For this review, take the finished solid that the model builds, in its own axes (mm). Give positions to 0.01 mm unless a question says otherwise; leave off trailing zeros. Loops run counter-clockwise (first coordinate to the right, second up) from the corner with the lowest first, then second, coordinate; pieces in that order, holes last.
```python
from build123d import *

# Parameters (mm, degrees)
BOARD_OUTLINE_DEPTH = 1.6
SKETCH2_R           = 1.016
SKETCH2_R_2         = 1.651
SKETCH2_R_3         = 0.254
SKETCH2_R_4         = 0.3
NPTH_DEPTH          = 55.024838732
SKETCH3_R           = 0.51
PTH_DEPTH           = 55.024838732
SKETCH4_W           = 11.674517828
SKETCH4_H           = 37.265337661
CUT_EXTRUDE1_DEPTH  = 10
SKETCH6_W           = 12.562793993
SKETCH6_H           = 36.934833376
CUT_EXTRUDE2_DEPTH  = 10


with BuildPart() as part:
    # Sketch1 → Board_Outline (new body)
    with BuildSketch(Plane.XY):
        Polygon((2.54, 35.56), (38.1, 35.56), (38.7574, 35.473452), (39.37, 35.219705), (39.896051, 34.816051), (40.299705, 34.29), (40.553452, 33.6774), (40.64, 33.02), (40.64, 2.54), (40.553452, 1.8826), (40.299705, 1.27), (39.896051, 0.743949), (39.37, 0.340295), (38.7574, 0.086548), (38.1, 0), (2.54, 0), (1.8826, 0.086548), (1.27, 0.340295), (0.743949, 0.743949), (0.340295, 1.27), (0.086548, 1.8826), (0, 2.54), (0, 33.02), (0.086548, 33.6774), (0.340295, 34.29), (0.743949, 34.816051), (1.27, 35.219705), (1.8826, 35.473452), align=None)
    extrude(amount=BOARD_OUTLINE_DEPTH)

    # Sketch2 → NPTH (cut, through all)
    with BuildSketch(Plane.XY):
        with Locations((20.32, 33.02)):
            Circle(SKETCH2_R)
        with Locations((20.32, 28.448)):
            Circle(SKETCH2_R)
        with Locations((2.54, 33.02)):
            Circle(SKETCH2_R_2)
        with Locations((38.1, 33.02)):
            Circle(SKETCH2_R_2)
        with Locations((2.54, 2.54)):
            Circle(SKETCH2_R_2)
        with Locations((38.1, 2.54)):
            Circle(SKETCH2_R_2)
        with Locations((21.463, 9.525)):
            Circle(SKETCH2_R_3)
        with Locations((27.686, 22.86)):
            Circle(SKETCH2_R_3)
        with Locations((20.955, 14.732)):
            Circle(SKETCH2_R_3)
        with Locations((24.13, 13.335)):
            Circle(SKETCH2_R_3)
        with Locations((24.13, 18.669)):
            Circle(SKETCH2_R_3)
        with Locations((19.304, 20.701)):
            Circle(SKETCH2_R_3)
        with Locations((18.415, 14.986)):
            Circle(SKETCH2_R_3)
        with Locations((16.383, 11.43)):
            Circle(SKETCH2_R_3)
        with Locations((16.571, 9.591)):
            Circle(SKETCH2_R_3)
        with Locations((26.67, 24.13)):
            Circle(SKETCH2_R_3)
        with Locations((26.543, 9.525)):
            Circle(SKETCH2_R_3)
        with Locations((26.924, 10.795)):
            Circle(SKETCH2_R_3)
        with Locations((26.289, 14.605)):
            Circle(SKETCH2_R_3)
        with Locations((21.463, 6.096)):
            Circle(SKETCH2_R_3)
        with Locations((14.605, 29.972)):
            Circle(SKETCH2_R_4)
        with Locations((21.209, 8.128)):
            Circle(SKETCH2_R_3)
        with Locations((27.305, 6.35)):
            Circle(SKETCH2_R_3)
        with Locations((27.432, 12.827)):
            Circle(SKETCH2_R_3)
        with Locations((21.844, 19.304)):
            Circle(SKETCH2_R_3)
        with Locations((21.844, 13.843)):
            Circle(SKETCH2_R_3)
        with Locations((25.4, 30.48)):
            Circle(SKETCH2_R_3)
        with Locations((22.86, 33.02)):
            Circle(SKETCH2_R_3)
    extrude(amount=NPTH_DEPTH, mode=Mode.SUBTRACT)

    # Sketch3 → PTH (cut, through all)
    with BuildSketch(Plane.XY):
        with Locations((11.43, 31.75)):
            Circle(SKETCH3_R)
        with Locations((11.43, 29.21)):
            Circle(SKETCH3_R)
        with Locations((11.43, 26.67)):
            Circle(SKETCH3_R)
        with Locations((34.29, 31.75)):
            Circle(SKETCH3_R)
        with Locations((11.43, 24.13)):
            Circle(SKETCH3_R)
        with Locations((11.43, 21.59)):
            Circle(SKETCH3_R)
        with Locations((11.43, 19.05)):
            Circle(SKETCH3_R)
        with Locations((11.43, 16.51)):
            Circle(SKETCH3_R)
        with Locations((11.43, 13.97)):
            Circle(SKETCH3_R)
        with Locations((11.43, 11.43)):
            Circle(SKETCH3_R)
        with Locations((11.43, 8.89)):
            Circle(SKETCH3_R)
        with Locations((11.43, 6.35)):
            Circle(SKETCH3_R)
        with Locations((11.43, 3.81)):
            Circle(SKETCH3_R)
        with Locations((29.21, 3.81)):
            Circle(SKETCH3_R)
        with Locations((29.21, 6.35)):
            Circle(SKETCH3_R)
        with Locations((29.21, 8.89)):
            Circle(SKETCH3_R)
        with Locations((29.21, 11.43)):
            Circle(SKETCH3_R)
        with Locations((29.21, 13.97)):
            Circle(SKETCH3_R)
        with Locations((29.21, 16.51)):
            Circle(SKETCH3_R)
        with Locations((29.21, 19.05)):
            Circle(SKETCH3_R)
        with Locations((29.21, 21.59)):
            Circle(SKETCH3_R)
        with Locations((29.21, 24.13)):
            Circle(SKETCH3_R)
        with Locations((29.21, 26.67)):
            Circle(SKETCH3_R)
        with Locations((29.21, 29.21)):
            Circle(SKETCH3_R)
        with Locations((29.21, 31.75)):
            Circle(SKETCH3_R)
        with Locations((6.35, 3.81)):
            Circle(SKETCH3_R)
        with Locations((6.35, 6.35)):
            Circle(SKETCH3_R)
        with Locations((6.35, 8.89)):
            Circle(SKETCH3_R)
        with Locations((6.35, 11.43)):
            Circle(SKETCH3_R)
        with Locations((6.35, 13.97)):
            Circle(SKETCH3_R)
        with Locations((6.35, 16.51)):
            Circle(SKETCH3_R)
        with Locations((34.29, 3.81)):
            Circle(SKETCH3_R)
        with Locations((34.29, 6.35)):
            Circle(SKETCH3_R)
        with Locations((34.29, 8.89)):
            Circle(SKETCH3_R)
        with Locations((34.29, 11.43)):
            Circle(SKETCH3_R)
        with Locations((34.29, 13.97)):
            Circle(SKETCH3_R)
        with Locations((34.29, 16.51)):
            Circle(SKETCH3_R)
        with Locations((34.29, 19.05)):
            Circle(SKETCH3_R)
        with Locations((34.29, 21.59)):
            Circle(SKETCH3_R)
        with Locations((6.35, 19.05)):
            Circle(SKETCH3_R)
        with Locations((6.35, 29.21)):
            Circle(SKETCH3_R)
        with Locations((34.29, 24.13)):
            Circle(SKETCH3_R)
        with Locations((34.29, 29.21)):
            Circle(SKETCH3_R)
        with Locations((6.35, 24.13)):
            Circle(SKETCH3_R)
        with Locations((6.35, 26.67)):
            Circle(SKETCH3_R)
        with Locations((34.29, 26.67)):
            Circle(SKETCH3_R)
        with Locations((6.35, 31.75)):
            Circle(SKETCH3_R)
        with Locations((6.35, 21.59)):
            Circle(SKETCH3_R)
    extrude(amount=PTH_DEPTH, mode=Mode.SUBTRACT)

    # Sketch4 → Cut-Extrude1 (cut)
    with BuildSketch(Plane.XY.offset(1.6)):
        with Locations((3.966399383, 16.92733117)):
            Rectangle(SKETCH4_W, SKETCH4_H)
    extrude(amount=-CUT_EXTRUDE1_DEPTH, mode=Mode.SUBTRACT)

    # Sketch6 → Cut-Extrude2 (cut)
    with BuildSketch(Plane(origin=(0, 0, 0), x_dir=(-1, 0, 0), z_dir=(0, 0, -1))):
        with Locations((-36.539437357, 18.467416688)):
            Rectangle(SKETCH6_W, SKETCH6_H)
    extrude(amount=-CUT_EXTRUDE2_DEPTH, mode=Mode.SUBTRACT)


solid = part.part
```
Item 1: The part is to be moulded in two halves that separate along X. For faces 1 (the flat face through (20, 18, 1.6)), 2 (the flat face through (30.258, 18, 1)), 3 (the cylindrical face through (29.1, 18.55, 0.79)), say which applies: released by +X, released by -X, zero draft, split by the parting line, or undercut.
Answer:
face 1: zero draft
face 2: released by +X
face 3: undercut
Item 2: For L1, parallel to Y at x = 20.32, z = 0.8; L2, parallel to X at y = 3.81, z = 0.85; L3, parallel to X at y = 33, z = 1.2, list the stretches that pass through material, from the lowest coordinate up.
Answer:
L1: y = 0 to 27.43, 29.46 to 32, 34.04 to 35.56
L2: x = 9.8 to 10.92, 11.94 to 28.7, 29.72 to 30.26
L3: x = 9.8 to 19.3, 21.34 to 22.61, 23.11 to 30.26
Item 3: Take a section at B-B on z = 1.1. State how many separate pieces and enclosed holes the cut face has, and give its area (3 significant figures).
Answer:
separate pieces: 1
enclosed holes: 48
area: 697 mm2
Item 4: Take a section at A-A on y = 26.67. Give the boundary of the cut face in (x, z).
Answer:
outline: (9.8, 0) - (10.92, 0) - (10.92, 1.6) - (9.8, 1.6) - close; (11.94, 0) - (28.7, 0) - (28.7, 1.6) - (11.94, 1.6) - close; (29.72, 0) - (30.26, 0) - (30.26, 1.6) - (29.72, 1.6) - close
